The drawing under review shows one solid part. Ordinate dimensions are in mm from its lowest x, y, z. Round coordinates to 2 decimals unless told otherwise and drop trailing zeros. Order: outer loops, then holes, each group sorted by start corner. A loop starts at its lowest first (then second) coordinate and runs counter-clockwise, first axis right, second up. Notation, with made-up numbers: M -36.75,-36 L 9.25,-36 A20 ccw 9.25,-29 Z; hole C 33,33 d11. An arc over 180 degrees is marked long. Answer as a JSON object with one key per item and string values.
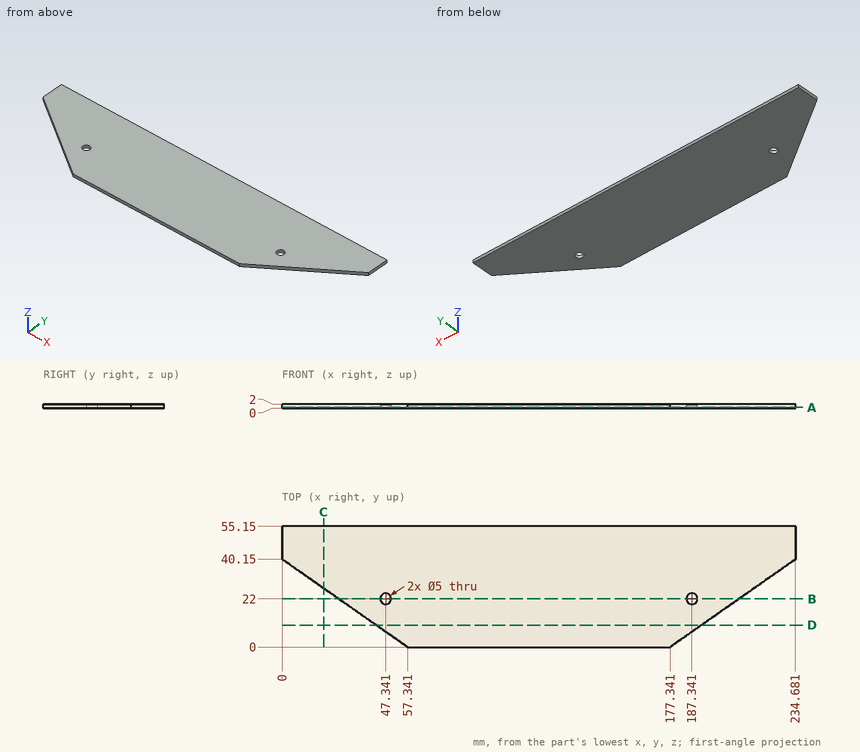
1) For L1, parallel to X at y = 20.5, z = 0.35 (1 decimal); L2, parallel to X at y = 6, z = 0.3; L3, parallel to Y at x = 46, z = 1.95, list the stretches that pass through material, from the lowest coordinate up.
Geometry check:
{"L1": "x = 28.1 to 45.3, 49.3 to 185.3, 189.3 to 206.6", "L2": "x = 48.77 to 185.91", "L3": "y = 7.94 to 19.89, 24.11 to 55.15"}
2) Add section D-D on y = 10. State the section outline as (x, z) points, and give its area (3 significant figures).
Geometry check:
{"outline": "M 43.06,0 L 191.62,0 L 191.62,2 L 43.06,2 Z", "area": "297 mm²"}
3) Add section C-C on x = 19. State the section outline as (y, z) points.
Geometry check:
{"outline": "M 26.85,0 L 55.15,0 L 55.15,2 L 26.85,2 Z"}
4) Add section B-B on y = 22. State the section outline as (x, z) points.
Geometry check:
{"outline": "M 25.92,0 L 44.84,0 L 44.84,2 L 25.92,2 Z; M 49.84,0 L 184.84,0 L 184.84,2 L 49.84,2 Z; M 189.84,0 L 208.76,0 L 208.76,2 L 189.84,2 Z"}
5) Add section A-A on z = 0.4. State the section outline as (x, y) points.
Geometry check:
{"outline": "M 0,40.15 L 57.34,0 L 177.34,0 L 234.68,40.15 L 234.68,55.15 L 0,55.15 Z; hole C 47.34,22 d5; hole C 187.34,22 d5"}
6) Insertion check: P1, Ø4.5, axis at x = 47.34, y = 22, coming from the -Z side. The pin has a flat end and moves straight along its axis. Give the tip position at first contact, or say it passes through.
Geometry check:
{"P1": "passes through"}
